Check sheet for the modelled part. Datum: model origin and axes. Units: mm. Face numbers are marked on the shaded views. A direction names the side the tool comes from. Round coordinates to 2 decimals unless told otherwise and drop trailing zeros. Write each loop counter-clockwise with the first axis right and the second up, starting at its lowest first coordinate (ties: lowest second). Pieces come first, ordered by that corner, then holes. Notation, with made-up numbers: (38, 50) -> (81, 50) arc R13 ccw to (81, 54) -> close; hole circle Ø4 at (62, 22.25). An arc over 180 degrees is marked (long way). Write item = value, one per line.
from build123d import *

# Parameters (mm, degrees)
BOSS_EXTRUDE2_DEPTH = 180
SKETCH3_W           = 23
SKETCH3_H           = 34
CUT_EXTRUDE2_DEPTH  = 10
SKETCH4_R           = 5.625
CUT_EXTRUDE3_DEPTH  = 10


with BuildPart() as part:
    # Sketch1 → Boss-Extrude2 (new body)
    with BuildSketch(Plane.XY):
        Polygon((0, 0), (40, 0), (40, -6), (6, -6), (6, -40), (0, -40), align=None)
    extrude(amount=-BOSS_EXTRUDE2_DEPTH)

    # Sketch3 → Cut-Extrude2 (cut)
    with BuildSketch(Plane(origin=(6, 0, 0), x_dir=(0, 0, -1), z_dir=(1, 0, 0))):
        with Locations((11.5, -23)):
            Rectangle(SKETCH3_W, SKETCH3_H)
        with Locations((168.5, -23)):
            Rectangle(SKETCH3_W, SKETCH3_H)
    extrude(amount=-CUT_EXTRUDE2_DEPTH, mode=Mode.SUBTRACT)

    # Sketch4 → Cut-Extrude3 (cut)
    with BuildSketch(Plane(origin=(0, 0, 0), x_dir=(1, 0, 0), z_dir=(0, 1, 0))):
        with Locations(Location((29.48, 142.4, 0), (0, 0, 270))):
            Circle(SKETCH4_R)
        with BuildLine():
            Line((34.98, 56.35), (34.98, 39.35))
            ThreePointArc((34.98, 39.35), (29.48, 33.85), (23.98, 39.35))
            Line((23.98, 39.35), (23.98, 56.35))
            ThreePointArc((23.98, 56.35), (29.48, 61.85), (34.98, 56.35))
        make_face()
    extrude(amount=-CUT_EXTRUDE3_DEPTH, mode=Mode.SUBTRACT)


solid = part.part
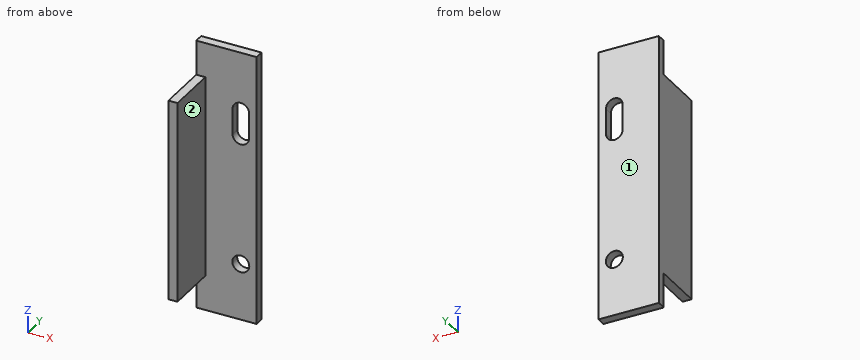
(1) Material ranges on L1, parallel to Z at x = 29, y = -4; L2, parallel to X at y = -2.4, z = -142.4 (3 decimals); L3, parallel to Y at x = 19.5, z = -39, recorded low to high. Write a range as [from, to].
Worked answers:
L1 = [-180, -148], [-136.8, -61.83], [-33.87, 0]
L2 = [0, 23.855], [35.105, 40]
L3 = [-6, 0]
(2) Sectioned sample at C-C on z = -48. Enter the section's corners in (x, y).
Worked answers:
outline = (0, -40) -> (6, -40) -> (6, -6) -> (23.98, -6) -> (23.98, 0) -> (0, 0) -> close; (34.98, -6) -> (40, -6) -> (40, 0) -> (34.98, 0) -> close
(3) Sectioned sample at B-B on z = -142.4. Enter the section's corners in (x, y) (3 decimals), then the cut area to 4 significant figures.
Worked answers:
outline = (0, -40) -> (6, -40) -> (6, -6) -> (23.855, -6) -> (23.855, 0) -> (0, 0) -> close; (35.105, -6) -> (40, -6) -> (40, 0) -> (35.105, 0) -> close
area = 376.5 mm²
(4) Access from +Z, -Z, +X, -X, +Y, -Y to the whole of each face (thin tool, end or side, straight path). Record for the marked faces 1 and 2.
Worked answers:
face_1 = +Z, -Z, +X, -X, +Y
face_2 = +Z, -Z, +X, -Y
(5) Sectioned sample at A-A on x = 29.48. Enter the section's corners in (y, z) (3 decimals), then the cut area to 4 significant figures.
Worked answers:
outline = (-6, -180) -> (0, -180) -> (0, -148.025) -> (-6, -148.025) -> close; (-6, -136.775) -> (0, -136.775) -> (0, -61.85) -> (-6, -61.85) -> close; (-6, -33.85) -> (0, -33.85) -> (0, 0) -> (-6, 0) -> close
area = 844.5 mm²
(6) Go/stop test with flat-tipped pins: P1, Ø10, axis at y = -15.5, z = -83, coming from the +X side; P2, Ø1, axis at x = 23, z = -49, coming from the -Y side; P3, Ø5, axis at x = 3, y = -29, coming from the +Z side. Record where each tip stops, or that it passes through.
Worked answers:
P1 = 6
P2 = -6
P3 = -23
(7) Sectioned sample at D-D on x = 16.5. Enter the section's corners in (y, z), then the cut area to 3 significant figures.
Worked answers:
outline = (-6, -180) -> (0, -180) -> (0, 0) -> (-6, 0) -> close
area = 1,080 mm²
